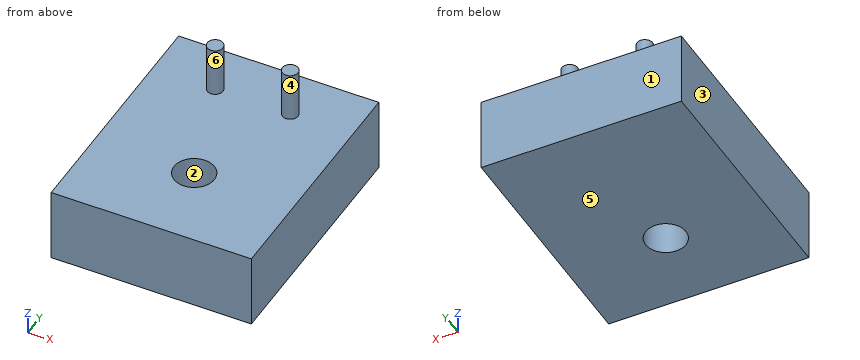
```python
from build123d import *

# Parameters (mm, degrees)
SKETCH1_W           = 25.4
SKETCH1_H           = 31.115
SKETCH1_R           = 2.5527
BOSS_EXTRUDE2_DEPTH = 9.525
SKETCH2_R           = 1
BOSS_EXTRUDE3_DEPTH = 6.35


with BuildPart() as part:
    # Sketch1 → Boss-Extrude2 (new body)
    with BuildSketch(Plane.XY):
        with Locations((12.7, -15.5575)):
            Rectangle(SKETCH1_W, SKETCH1_H)
        with Locations((12.7, -20.6375)):
            Circle(SKETCH1_R, mode=Mode.SUBTRACT)
    extrude(amount=BOSS_EXTRUDE2_DEPTH)

    # Sketch2 → Boss-Extrude3 (add)
    with BuildSketch(Plane.XY.offset(9.525)):
        with Locations((7.9375, -6.35)):
            Circle(SKETCH2_R)
        with Locations((17.4625, -6.35)):
            Circle(SKETCH2_R)
    extrude(amount=BOSS_EXTRUDE3_DEPTH)


solid = part.part
```
Work out the finished part from the listing and answer in its coordinate system (mm). Face numbers are marked on the shaded views. A direction names the side the tool comes from. Give positions to 0.01 mm unless a question says otherwise; leave off trailing zeros. Order: outer loops, then holes, each group sorted by start corner. A loop starts at its lowest first (then second) coordinate and runs counter-clockwise, first axis right, second up. Notation, with made-up numbers: (-38, 35) -> (4, 35) arc R25 ccw to (4, 67) -> close; hole circle Ø10 at (67, 6). An arc over 180 degrees is marked (long way). Answer as CSV lines item,"result". Start each with the question number.
(1) Which of the six approach directions +Z, -Z, +X, -X, +Y, -Y give full straight-line access (tool end or side, diameter ignored) to the marked faces 5 and 6?
(2) Section D-D, the plane y = -6.35 is taken. Write down the section's boundary in (x, z) (1 decimal), plus the area to 3 significant figures.
(3) Consider line 1 along Y through (x, z) = (12.7, 4.5) (3 decimals); line 2 along Y through (x, z) = (11.75, 6.25) (3 decimals); line 3 along Z through (x, y) = (19.75, -8) (3 decimals). Determine where each line is inside the solid, lowest interval first.
(4) Section B-B, the plane y = -21.5 is taken. Write down the section's boundary in (x, z) (3 decimals).
(5) Each of these flat-tipped pins is pushed along its axis until it touches: pin 1 Ø3 at (x, y) = (5, -11) entering from +Z (3 decimals); pin 2 Ø2 at (x, z) = (12.5, 6) entering from +Y. Where does it stop, or does it pass through?
(6) For a pull along X with two mould halves and no side action, classify the marked faces 1, 2, 3 and 4 as released by +X, released by -X, zero draft, split by the parting line, or undercut.
(7) Section A-A, the plane x = 12.7 is taken. Write down the section's boundary in (y, z) (3 decimals).
(8) Section C-C, the plane z = 10.25 is taken. Write down the section's boundary in (x, y), plus the area to 3 significant figures.
Entries:
1,face 5,"-Z, +X, -X, +Y, -Y"
1,face 6,"+Z"
2,outline,"(0, 0) -> (25.4, 0) -> (25.4, 9.5) -> (18.5, 9.5) -> (18.5, 15.9) -> (16.5, 15.9) -> (16.5, 9.5) -> (8.9, 9.5) -> (8.9, 15.9) -> (6.9, 15.9) -> (6.9, 9.5) -> (0, 9.5) -> close"
2,area,"267 mm²"
3,line 1,"-31.115 to -23.19, -18.085 to 0"
3,line 2,"-31.115 to -23.007, -18.268 to 0"
3,line 3,"0 to 9.525"
4,outline,"(0, 0) -> (10.297, 0) -> (10.297, 9.525) -> (0, 9.525) -> close; (15.103, 0) -> (25.4, 0) -> (25.4, 9.525) -> (15.103, 9.525) -> close"
5,pin 1,"z = 9.525"
5,pin 2,"y = 0"
6,face 1,"zero draft"
6,face 2,"undercut"
6,face 3,"released by -X"
6,face 4,"undercut"
7,outline,"(-31.115, 0) -> (-23.19, 0) -> (-23.19, 9.525) -> (-31.115, 9.525) -> close; (-18.085, 0) -> (0, 0) -> (0, 9.525) -> (-18.085, 9.525) -> close"
8,outline,"circle Ø2 at (7.94, -6.35); circle Ø2 at (17.46, -6.35)"
8,area,"6.28 mm²"
